Autodesk Inventor part; units mm, degrees
ref_plane "YZ Plane" through (0, 0, 0) normal (1, 0, 0) x (0, 1, 0)
ref_plane "XZ Plane" through (0, 0, 0) normal (0, 1, 0) x (-1, 0, 0)
ref_plane "XY Plane" through (0, 0, 0) normal (0, 0, 1) x (1, 0, 0)
sketch "Sketch1" plane through (0, 0, 0) normal (0, 1, 0) x (-1, 0, 0)
  circle A0 centre (0, 0) radius 1.95
  dimension "d0" = 3.9
extrude "Extrusion1" add sketch "Sketch1" along normal blind 15.8
sketch "Sketch2" plane through (0, 15.8, 0) normal (0, 1, 0) x (1, 0, 0)
  circle A0 centre (0, 0) radius 3.5
  dimension "d3" = 7
extrude "Extrusion2" add sketch "Sketch2" along normal blind 2.7
sketch "Sketch3" plane through (0, 18.5, 0) normal (0, 1, 0) x (1, 0, 0)
  line L0 (0.75, -8) -> (-0.75, -8)
  line L1 (-0.75, -8) -> (-0.75, 8)
  line L2 (-0.75, 8) -> (0.75, 8)
  line L3 (0.75, 8) -> (0.75, -8)
  line L4 (0.75, -8) -> (-0.75, 8) construction
  line L5 (-0.75, -8) -> (0.75, 8) construction
  point P0 (0, 0)
  dimension "d6" = 1.5
  dimension "d7" = 16
extrude "Extrusion3" cut sketch "Sketch3" against normal blind 1.5
properties part number "screw18.5mm" material "Stainless Steel"
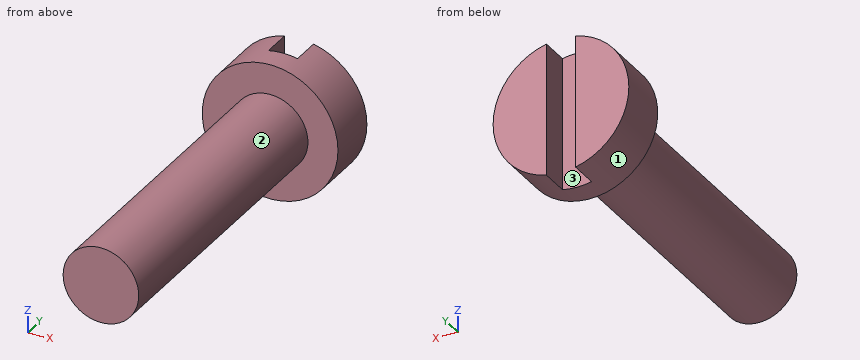
Geometry check sheet. Reference: the model listing, model coordinates, mm. Face numbers are marked on the shaded views. A direction names the side the tool comes from. Round coordinates to 2 decimals unless told otherwise and drop trailing zeros. Order: outer loops, then holes, each group sorted by start corner. A loop starts at its lowest first (then second) coordinate and runs counter-clockwise, first axis right, second up. Notation, with made-up numbers: (73.5, -30) -> (85.5, -30) arc R17 cw to (85.5, -22) -> close; hole circle Ø1 at (-33, 50). An arc over 180 degrees is marked (long way). Return JSON: item names as keys, results as strings. Group by question number.
Q1. Gauge pin test, flat ends, axial feed: pin 1 (3 mm diameter, centred on x = 2.5, y = 11, fed in from +Z); pin 2 (3 mm diameter, centred on y = 6, z = 0, fed in from +X); pin 3 (0.8 mm diameter, centred on x = 0, z = -1.5, fed in from +Y). Record the tip position at first contact, or that the pin passes through.
Q2. Section check B-B, the plane x = 0. Record the boundary of the cut face in (y, z).
Q3. Tool access check on the marked faces 1, 2 and 3. Record the directions out of +Z, -Z, +X, -X, +Y, -Y that give a thin tool (end or side, any length) a straight path to the whole face; none if there is none.
Q4. Material ranges on probe 1 along Z at (x, y) = (0, 15); probe 2 along Y at (x, z) = (2.25, 0.75); probe 3 along Y at (x, z) = (0.25, -2.25), recorded low to high. Write a range as from..to.
Q5. Section check A-A, the plane z = 0. Record the boundary of the cut face in (x, y).
Q6. Section check D-D, the plane y = 14. Record the boundary of the cut face in (x, z), plus the area to 3 significant figures.
Q7. Section check C-C, the plane y = 17.5. Record the boundary of the cut face in (x, z), plus the area to 3 significant figures.
Numbers:
{
 "1": {"pin 1": "z = 1.67", "pin 2": "x = 1.95", "pin 3": "y = 17"},
 "2": {"outline": "(0, -1.95) -> (15.8, -1.95) -> (15.8, -3.5) -> (17, -3.5) -> (17, 3.5) -> (15.8, 3.5) -> (15.8, 1.95) -> (0, 1.95) -> close"},
 "3": {"face 1": "+Y, -Y", "face 2": "-Y", "face 3": "+Z, -Z, +Y"},
 "4": {"probe 1": "-1.95..1.95", "probe 2": "15.8..18.5", "probe 3": "15.8..17"},
 "5": {"outline": "(-3.5, 15.8) -> (-1.95, 15.8) -> (-1.95, 0) -> (1.95, 0) -> (1.95, 15.8) -> (3.5, 15.8) -> (3.5, 18.5) -> (0.75, 18.5) -> (0.75, 17) -> (-0.75, 17) -> (-0.75, 18.5) -> (-3.5, 18.5) -> close"},
 "6": {"outline": "circle Ø3.9 at (0, 0)", "area": "11.9 mm^2"},
 "7": {"outline": "(-0.75, -3.42) -> (-0.75, 3.42) arc R3.5 ccw to start; (0.75, -3.42) arc R3.5 ccw to (0.75, 3.42) -> close", "area": "28.1 mm^2"}
}
